Print and shaded views of the part. All mm, measured from the part's lowest x, y and z. Round coordinates to 2 decimals unless told otherwise and drop trailing zeros. Order: outer loops, then holes, each group sorted by start corner. A loop starts at its lowest first (then second) coordinate and runs counter-clockwise, first axis right, second up. Notation, with made-up numbers: M 7.25,66.5 L 59.25,66.5 A23 cw 59.25,76.5 Z; hole C -25,82 d4. An arc over 180 degrees is marked long. Use CSV: the item, a comma, the result in double quotes.
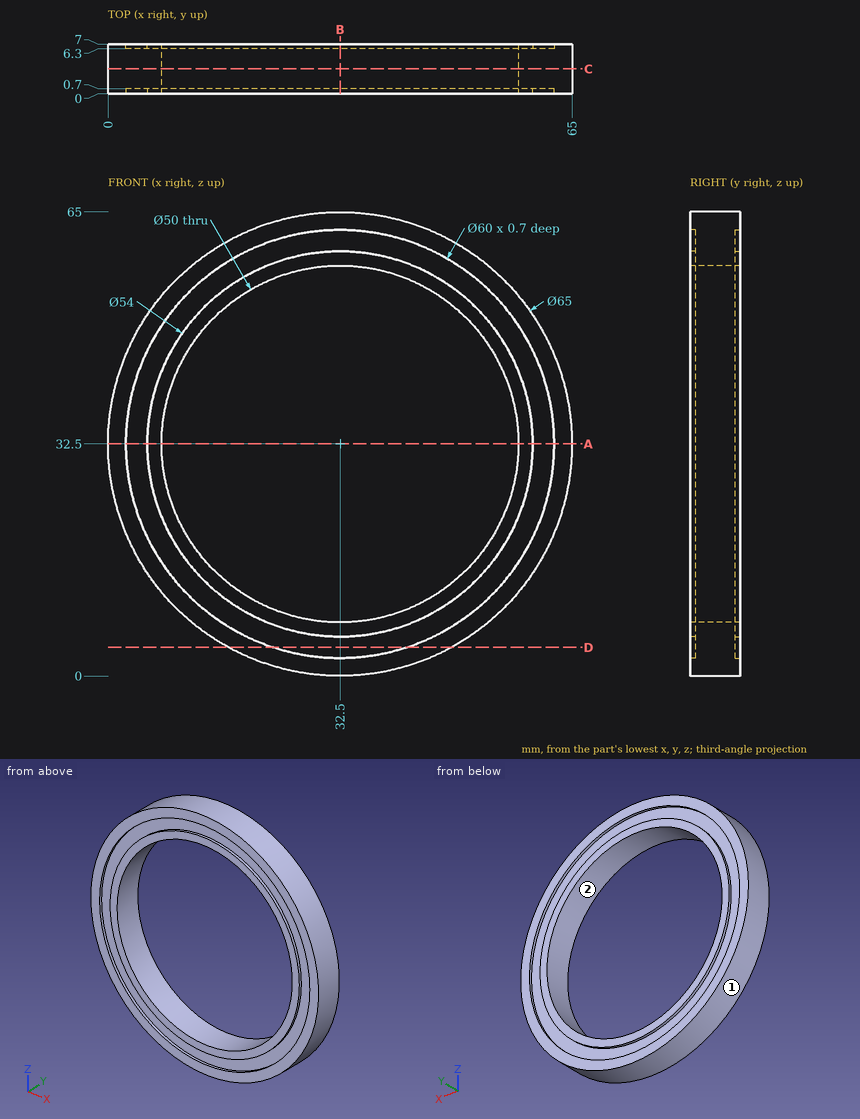
(1) Two-plate mould, pull along X, no slides. Class the marked faces 1 and 2: released by +X, released by -X, zero draft, split by the parting line, or undercut.
Answer block:
face 1,"split by the parting line"
face 2,"undercut"
(2) Cut at A-A, the plane z = 32.5. Give the cut face in (x, y), and give its area (3 significant figures).
Answer block:
outline,"M 0,0 L 2.5,0 L 2.5,0.7 L 5.5,0.7 L 5.5,0 L 7.5,0 L 7.5,7 L 5.5,7 L 5.5,6.3 L 2.5,6.3 L 2.5,7 L 0,7 Z; M 57.5,0 L 59.5,0 L 59.5,0.7 L 62.5,0.7 L 62.5,0 L 65,0 L 65,7 L 62.5,7 L 62.5,6.3 L 59.5,6.3 L 59.5,7 L 57.5,7 Z"
area,"96.6 mm²"
(3) Wall check: line 1 (Z direction, x = 32.5, y = 6.5); line 2 (Z direction, x = 32.5, y = 1.75); line 3 (X direction, y = 0.75, z = 45.5). Give the ranges that are in metal, low to high. Write a range as from..to.
Answer block:
line 1,"z = 0..2.5, 5.5..7.5, 57.5..59.5, 62.5..65"
line 2,"z = 0..7.5, 57.5..65"
line 3,"x = 2.71..11.15, 53.85..62.29"
(4) Cut at B-B, the plane x = 32.5. Give the cut face in (y, z), and give its area (3 significant figures).
Answer block:
outline,"M 0,0 L 7,0 L 7,2.5 L 6.3,2.5 L 6.3,5.5 L 7,5.5 L 7,7.5 L 0,7.5 L 0,5.5 L 0.7,5.5 L 0.7,2.5 L 0,2.5 Z; M 0,57.5 L 7,57.5 L 7,59.5 L 6.3,59.5 L 6.3,62.5 L 7,62.5 L 7,65 L 0,65 L 0,62.5 L 0.7,62.5 L 0.7,59.5 L 0,59.5 Z"
area,"96.6 mm²"
(5) Cut at D-D, the plane z = 4. Give the cut face in (x, y), and give its area (3 significant figures).
Answer block:
outline,"M 16.88,0 L 23.13,0 L 23.13,0.7 L 41.87,0.7 L 41.87,0 L 48.12,0 L 48.12,7 L 41.87,7 L 41.87,6.3 L 23.13,6.3 L 23.13,7 L 16.88,7 Z"
area,"192 mm²"
(6) Drop a flat-ended pin along its axis: pin 1 (2 mm diameter, centred on y = 2, z = 48.5, fed in from -X). Give the stop position or say it passes through.
Answer block:
pin 1,"stops at x = 3.67"
(7) Cut at C-C, the plane y = 3.5. Give the cut face in (x, z), and give its area (3 significant figures).
Answer block:
outline,"C 32.5,32.5 d65; hole C 32.5,32.5 d50"
area,"1,350 mm²"
